CAD build for the part. Positions are in the model's coordinates, mm. A direction names the side the tool comes from. Round coordinates to 2 decimals unless told otherwise and drop trailing zeros. Loops run counter-clockwise (first coordinate to the right, second up) from the corner with the lowest first, then second, coordinate; pieces in that order, holes last. Notation, with made-up numbers: M 69,13 L 76,13 A10 ccw 76,22 Z; hole C 4.25,-22.75 d7. An arc over 180 degrees is marked long. Use a Markdown table: item, result. Add a question column.
(1) Flat gauge pins, fed straight in: P1, Ø12.5, axis at x = 44, y = -17, coming from the +Z side; P2, Ø1, axis at x = 16.5, z = 12, coming from the +Y side. Where does each tip first touch, or does it go through?
(2) Band-saw the part on D-D, the plane y = -10. Write the cut outline in (x, z).
(3) Band-saw the part on C-C, the plane x = 9.5. Write the cut outline in (y, z).
(4) Two-plate mould, pull along Y, no slides. Class faces 4 (the face through (22, 0, 10)), 5 (the face through (6, -6.35, 38)), 6 (the face through (6.261, -23.745, 39.721)): released by +Y, released by -Y, zero draft, split by the parting line, or undercut.
(5) Band-saw the part on A-A, the plane y = -12.7. Write the cut outline in (x, z).
(6) Which spindle directions (+Z, -Z, +X, -X, +Y, -Y) get a long thin tool onto all of the face, cutting with end or side? Do faces 1 (the face through (57.15, -13, 6)), 2 (the face through (6, -19.05, 38)), 3 (the face through (35, -13, 12.7)). Say none if no direction does.
(7) Wall check: L1, parallel to Y at x = 3, z = 31.5; L2, parallel to Z at x = 27, y = -4.75. Give the ranges that are in metal, low to high.
(8) Band-saw the part on B-B, the plane x = 44.45. Write the cut outline in (y, z).
from build123d import *

# Parameters (mm, degrees)
F0_W        = 57.15
F0_H        = 44.45
F1_DEPTH    = 25.4
F2_W        = 44.45
F2_H        = 31.75
F3_DEPTH    = 25.4
F4_R        = 6.35
F5_DEPTH    = 25.4
F7_DEPTH    = 25.4
F8_T1_DEPTH = 67.6926131403


# Not quite as in the source:
# - a fillet or chamfer that OpenCascade refuses, or shapes differently, is made with other operations: its cross-section is extruded or revolved along the edge and cut away or added


with BuildPart() as f1:
    # F0 (on Front) → F1 (new body)
    with BuildSketch(Plane.XZ):
        with Locations((28.575, 22.225)):
            Rectangle(F0_W, F0_H)
    extrude(amount=F1_DEPTH)

    # F2 (on face) → F3 (cut)
    with BuildSketch(Plane.XZ.offset(25.4)):
        with Locations((34.925, 28.575)):
            Rectangle(F2_W, F2_H)
    extrude(amount=-F3_DEPTH, mode=Mode.SUBTRACT)

    # F4 (on face) → F5 (cut)
    with BuildSketch(Plane.XY.offset(12.7)):
        with Locations((25.4, -12.7)):
            Circle(F4_R)
        with Locations((44.45, -12.7)):
            Circle(F4_R)
    extrude(amount=-F5_DEPTH, mode=Mode.SUBTRACT)

    # F6 (on face) → F7 (cut)
    with BuildSketch(Plane.YZ.offset(12.7)):
        with BuildLine():
            ThreePointArc((-19.05, 31.75), (-12.7, 38.1), (-6.35, 31.75))
            Line((-6.35, 31.75), (-6.35, 44.45))
            Line((-6.35, 44.45), (-19.05, 44.45))
            Line((-19.05, 44.45), (-19.05, 31.75))
        make_face()
        with BuildLine():
            ThreePointArc((-19.05, 31.75), (-12.7, 25.4), (-6.35, 31.75))
            ThreePointArc((-6.35, 31.75), (-12.7, 38.1), (-19.05, 31.75))
        make_face()
    extrude(amount=-F7_DEPTH, mode=Mode.SUBTRACT)

    # F8: fillet of radius 12.7 on 2 edges, made by hand

    # F8_s2 → F8_t1 (cut)
    with BuildSketch(Plane.YZ.offset(-27.4963065702)):
        with BuildLine():
            ThreePointArc((-25.4, 33.4514773719), (-23.6985226281, 39.8014773719), (-19.05, 44.45))
            Line((-19.05, 44.45), (-25.4, 44.45))
            Line((-25.4, 44.45), (-25.4, 33.4514773719))
        make_face()
        with BuildLine():
            ThreePointArc((0, 33.4514773719), (-1.7014773719, 39.8014773719), (-6.35, 44.45))
            Line((-6.35, 44.45), (0, 44.45))
            Line((0, 44.45), (0, 33.4514773719))
        make_face()
    extrude(amount=F8_T1_DEPTH, mode=Mode.SUBTRACT)


solid = f1.part
Return value:
| question | item | result |
|---|---|---|
| 1 | P1 | z = 12.7 |
| 1 | P2 | y = 0 |
| 2 | outline | M 0,0 L 19.65,0 L 19.65,12.7 L 12.7,12.7 L 12.7,26 L 0,26 Z; M 31.15,0 L 38.7,0 L 38.7,12.7 L 31.15,12.7 Z; M 50.2,0 L 57.15,0 L 57.15,12.7 L 50.2,12.7 Z |
| 3 | outline | M -25.4,0 L 0,0 L 0,33.45 A12.7 ccw -6.35,44.45 L -6.35,31.75 A6.35 cw -19.05,31.75 L -19.05,44.45 A12.7 ccw -25.4,33.45 Z |
| 4 | face 4 | released by +Y |
| 4 | face 5 | undercut |
| 4 | face 6 | released by -Y |
| 5 | outline | M 0,0 L 19.05,0 L 19.05,12.7 L 12.7,12.7 L 12.7,25.4 L 0,25.4 Z; M 31.75,0 L 38.1,0 L 38.1,12.7 L 31.75,12.7 Z; M 50.8,0 L 57.15,0 L 57.15,12.7 L 50.8,12.7 Z |
| 6 | face 1 | +Z, -Z, +X, +Y, -Y |
| 6 | face 2 | +Z, +X, -X |
| 6 | face 3 | +Z, +X, +Y, -Y |
| 7 | L1 | -25.4 to -19.05, -6.35 to 0 |
| 7 | L2 | 0 to 12.7 |
| 8 | outline | M -25.4,0 L -19.05,0 L -19.05,12.7 L -25.4,12.7 Z; M -6.35,0 L 0,0 L 0,12.7 L -6.35,12.7 Z |
